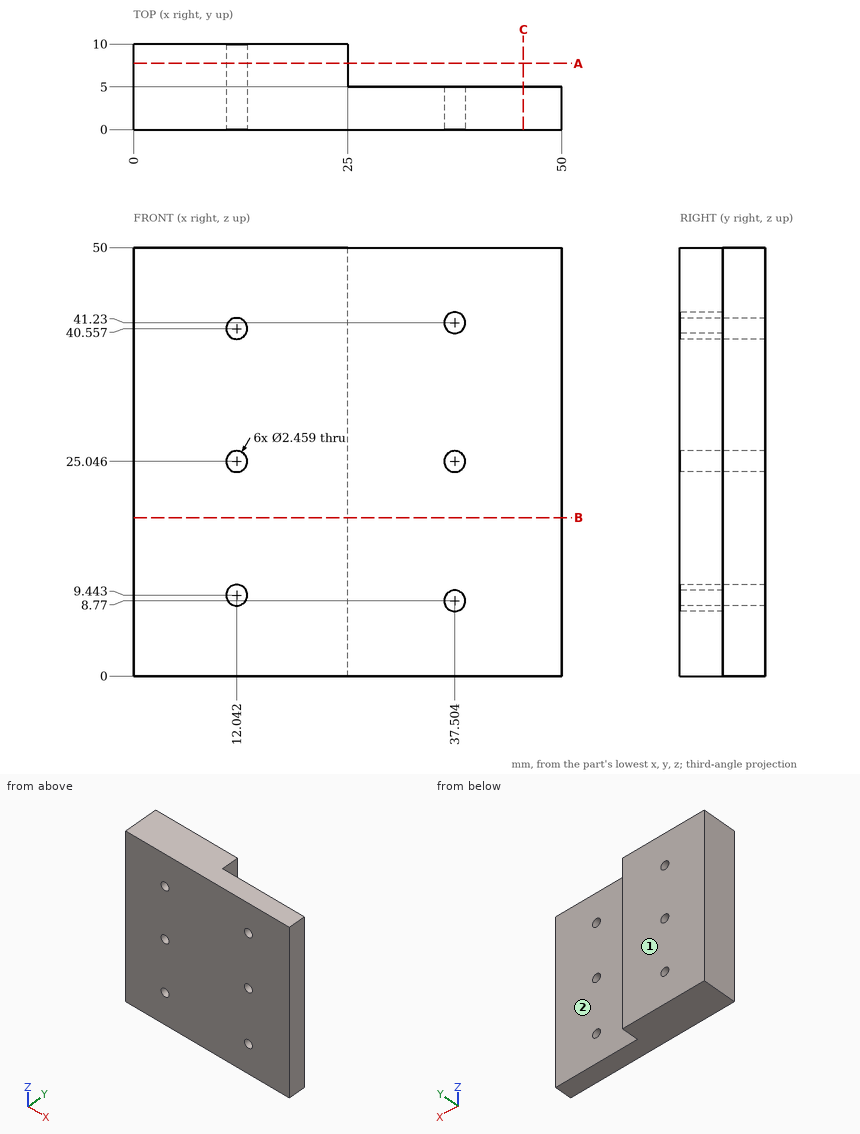
Geometry check sheet. Reference: drawing and pictorial views, mm from the part's lowest x, y, z. A direction names the side the tool comes from. Give positions to 0.01 mm unless a question says otherwise; leave off trailing zeros. Order: outer loops, then holes, each group sorted by start corner. A loop starts at its lowest first (then second) coordinate and runs counter-clockwise, first axis right, second up. Notation, with made-up numbers: M -12,41 L 21,41 A17 cw 21,62 Z; hole C -27,-18 d6. An arc over 180 degrees is marked long. Use one line per item in the form item = value. Start each with the question number.
Q1. Section check B-B (z = 18.5). Enter the section's corners in (x, y), then the cut area to 3 significant figures.
Q2. Section check A-A (y = 7.75). Enter the section's corners in (x, z) (1 decimal).
Q3. Section check C-C (x = 45.5). Enter the section's corners in (y, z).
Q4. Go/stop test with flat-tipped pins: pin 1 Ø2.5 at (y, z) = (6.5, 26) entering from +X; pin 2 Ø3 at (x, z) = (37.5, 25.05) entering from +Y. Record where each tip stops, or that it passes through.
Q5. Access from +Z, -Z, +X, -X, +Y, -Y to the whole of each face (thin tool, end or side, straight path). Record for the marked faces 1 and 2.
Q6. Scan lines: line 1 along X through (y, z) = (4.75, 25) (1 decimal); line 2 along X through (y, z) = (7.25, 34); line 3 along X through (y, z) = (6.75, 40) (1 decimal). Record each from-to range of solid material in increasing order. Write a range as [from, to].
Evaluation:
q1.outline = M 0,0 L 50,0 L 50,5 L 25,5 L 25,10 L 0,10 Z
q1.area = 375 mm2
q2.outline = M 0,0 L 25,0 L 25,50 L 0,50 Z; hole C 12,9.4 d2.5; hole C 12,25 d2.5; hole C 12,40.6 d2.5
q3.outline = M 0,0 L 5,0 L 5,50 L 0,50 Z
q4.pin_1 = 25
q4.pin_2 = 5
q5.face_1 = +Z, -Z, +X, -X, +Y
q5.face_2 = +Z, -Z, +X, +Y
q6.line_1 = [0, 10.8], [13.3, 36.3], [38.7, 50]
q6.line_2 = [0, 25]
q6.line_3 = [0, 10.9], [13.1, 25]
